```python
from build123d import *

# Parameters (mm, degrees)
BOSS_EXTRUDE1_DEPTH      = 152.4
BOSS_EXTRUDE1_DEPTH_BACK = 152.4
SKETCH4_R                = 1.5875
CUT_EXTRUDE1_DEPTH       = 1.5875
SKETCH5_R                = 3.175
CUT_EXTRUDE2_DEPTH       = 1.5875


with BuildPart() as part:
    # Sketch3 → Boss-Extrude1 (new, two sides: drawn at the far end of the back side and taken through both)
    with BuildSketch(Plane.XY.offset(-BOSS_EXTRUDE1_DEPTH_BACK)):
        Polygon((30.95625, -14.2875), (30.95625, -15.875), (-0.79375, -15.875), (-0.79375, 14.2875), (-16.66875, 14.2875), (-16.66875, 15.875), (0.79375, 15.875), (0.79375, -14.2875), align=None)
    extrude(amount=BOSS_EXTRUDE1_DEPTH + BOSS_EXTRUDE1_DEPTH_BACK)

    # Sketch4 → Cut-Extrude1 (cut)
    with BuildSketch(Plane(origin=(0, -14.2875, 0), x_dir=(1, 0, 0), z_dir=(0, 1, 0))):
        with Locations(Location((15.875, 27.94, 0), (0, 0, 270))):
            Circle(SKETCH4_R)
        with Locations(Location((15.875, -48.26, 0), (0, 0, 270))):
            Circle(SKETCH4_R)
        with Locations(Location((15.875, -124.46, 0), (0, 0, 270))):
            Circle(SKETCH4_R)
    extrude(amount=-CUT_EXTRUDE1_DEPTH, mode=Mode.SUBTRACT)

    # Sketch5 → Cut-Extrude2 (cut)
    with BuildSketch(Plane(origin=(0.79375, 0, 0), x_dir=(0, 0, -1), z_dir=(1, 0, 0))):
        with Locations((-138.4808, 0.79375)):
            Circle(SKETCH5_R)
        with Locations((146.05, 0.79375)):
            Circle(SKETCH5_R)
    extrude(amount=-CUT_EXTRUDE2_DEPTH, mode=Mode.SUBTRACT)


solid = part.part
```
CAD build for the part. Positions are in the model's coordinates, mm. A direction names the side the tool comes from. Give positions to 0.01 mm unless a question says otherwise; leave off trailing zeros. Order: outer loops, then holes, each group sorted by start corner. A loop starts at its lowest first (then second) coordinate and runs counter-clockwise, first axis right, second up.
(1) Saw through at D-D, the plane y = 7. Give the cut face in (x, z), then the cut area to 3 significant figures.
(2) Saw through at B-B, the plane z = 58.5. Give the cut face in (x, y) (1 decimal), then the cut area to 3 significant figures.
(3) Flat gauge pins, fed straight in: pin 1 (5 mm diameter, centred on x = 15.875, z = 48.26, fed in from -Y) (3 decimals); pin 2 (24 mm diameter, centred on x = 13.5, z = -0.5, fed in from +Y); pin 3 (6 mm diameter, centred on x = -9.5, z = 102.5, fed in from -Y); pin 4 (5 mm diameter, centred on y = -5, z = -112, fed in from -X). Where does each tip first touch, or does it go through?
(4) Saw through at C-C, the plane x = 11. Give the cut face in (y, z) (1 decimal), then the cut area to 3 significant figures.
(5) Drill centre lines: L1, parallel to X at y = -14.9, z = -27.94; L2, parallel to X at y = -15, z = 48; L3, parallel to X at y = -14, z = -11. Where is each one in solid material? Low to high.
(6) Mould opens along Y. For faces 4 (the flat face through (-8, 15.875, -2)), 5 (the flat face through (15, -15.875, -2)), 6 (the cylindrical face through (0.011, -0.422, -148.983)), 7 (the cylindrical face through (0.011, 0.933, 141.653)) say: released by +Y, released by -Y, zero draft, split by the parting line, or undercut.
(7) Saw through at A-A, the plane z = -146.05. Give the cut face in (x, y) (1 decimal), then the cut area to 3 significant figures.
(8) Tool access for faces 1 (the flat face through (0, -2, -152.4)), 2 (the flat face through (-9, 14.288, -2)), 3 (the flat face through (16, -14.288, -2)): list every direction of +Z, -Z, +X, -X, +Y, -Y with a clear straight run to the whole face (end or side of a thin tool).
Results found:
1. outline: (-0.79, -152.4) - (0.79, -152.4) - (0.79, 152.4) - (-0.79, 152.4) - close
1. area: 484 mm2
2. outline: (-16.7, 14.3) - (-0.8, 14.3) - (-0.8, -15.9) - (31, -15.9) - (31, -14.3) - (0.8, -14.3) - (0.8, 15.9) - (-16.7, 15.9) - close
2. area: 123 mm2
3. pin 1: stops at y = -15.875
3. pin 2: stops at y = -14.29
3. pin 3: stops at y = 14.29
3. pin 4: stops at x = -0.79
4. outline: (-15.9, -152.4) - (-14.3, -152.4) - (-14.3, 152.4) - (-15.9, 152.4) - close
4. area: 484 mm2
5. L1: x = -0.79 to 14.29, 17.46 to 30.96
5. L2: x = -0.79 to 14.31, 17.44 to 30.96
5. L3: x = -0.79 to 0.79
6. face 4: released by +Y
6. face 5: released by -Y
6. face 6: undercut
6. face 7: undercut
7. outline: (-16.7, 14.3) - (-0.8, 14.3) - (-0.8, 4) - (0.8, 4) - (0.8, 15.9) - (-16.7, 15.9) - close; (-0.8, -15.9) - (31, -15.9) - (31, -14.3) - (0.8, -14.3) - (0.8, -2.4) - (-0.8, -2.4) - close
7. area: 113 mm2
8. face 1: -Z, +X, -X, +Y, -Y
8. face 2: +Z, -Z, -X, -Y
8. face 3: +Z, -Z, +X, +Y
